Here's the drawing with two shaded views (mm, measured from the low corner). I have some questions. A direction names the side the tool comes from. Coordinates: 2 decimals unless noted, no trailing zeros. Write each loop counter-clockwise with the first axis right and the second up, starting at its lowest first coordinate (ties: lowest second). Pieces come first, ordered by that corner, then holes. Notation, with made-up numbers: M 28,75.25 L 53,75.25 A18 cw 53,96.25 Z; hole C 32.5,67 d6. An arc over 180 degrees is marked long. Answer as CSV lines item,"result". Start each with the question number.
Item 1: Suppose I cut it at B-B, the plane x = 2.5. Write out the boundary of the cut face in (y, z), and give its area (3 significant figures).
Item 2: Suppose I cut it at C-C, the plane z = 5.5. Write out the boundary of the cut face in (x, y), and give its area (3 significant figures).
Item 3: I'm going to push flat-ended pins straight in: P1, Ø1.5, axis at x = 2, z = 11.5, coming from the +Y side; P2, Ø5.5, axis at x = 7.5, y = 13, coming from the +Z side; P3, Ø5.5, axis at y = 13, z = 17, coming from the -X side. Where does each tip first touch, or does it pass through?
Item 4: Suppose I cut it at A-A, the plane y = 12.5. Write out the boundary of the cut face in (x, z), and give its area (3 significant figures).
Item 5: Suppose I cut it at D-D, the plane y = 9.5. Write out the boundary of the cut face in (x, z).
Item 6: We'd pull the mould along X, two halves only. Please class the marked faces 1, 2, 3 and 4: +X half, -X half, draft (parallel to the pull), parting line (faces both ways), or undercut.
Item 7: If I drill on line 1 along Y through (x, z) = (6.5, 20); line 2 along Z through (x, y) = (9.5, 12.5); line 3 along Z through (x, y) = (1.5, 11.25), over which ranges is the centre line in solid material (lowest first)? Write a range as [from, to].
Item 8: On a 3-axis mill with a long thin cutter (end or side, diameter ignored), from which of +Z, -Z, +X, -X, +Y, -Y can I reach the whole of each face in a straight line? I mean the marked faces 5, 6 and 7. Say none if no direction works.
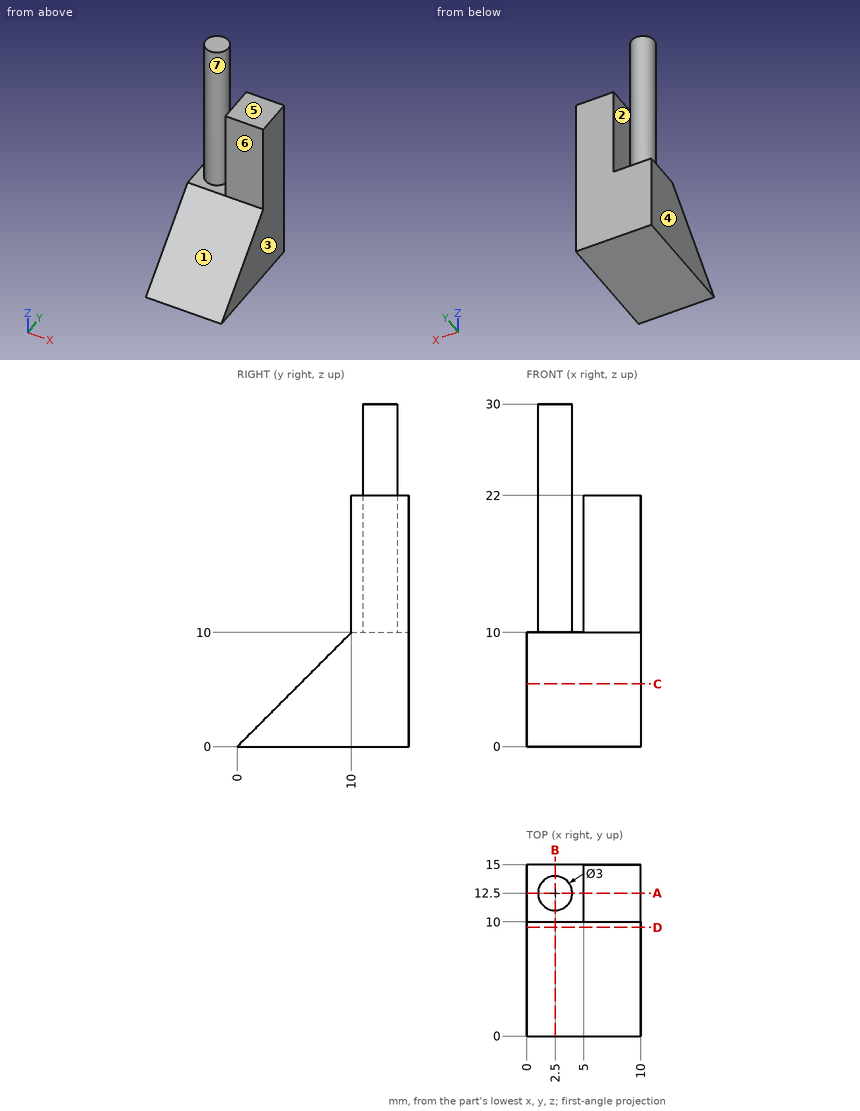
Ans:
1,outline,"M 0,0 L 15,0 L 15,10 L 14,10 L 14,30 L 11,30 L 11,10 L 10,10 Z"
1,area,"160 mm^2"
2,outline,"M 0,5.5 L 10,5.5 L 10,15 L 0,15 Z"
2,area,"95.0 mm^2"
3,P1,"stops at y = 14"
3,P2,"stops at z = 22"
3,P3,"stops at x = 1"
4,outline,"M 0,0 L 10,0 L 10,22 L 5,22 L 5,10 L 4,10 L 4,30 L 1,30 L 1,10 L 0,10 Z"
4,area,"220 mm^2"
5,outline,"M 0,0 L 10,0 L 10,9.5 L 0,9.5 Z"
6,face 1,"draft"
6,face 2,"undercut"
6,face 3,"+X half"
6,face 4,"-X half"
7,line 1,"y = [10, 15]"
7,line 2,"z = [0, 22]"
7,line 3,"z = [0, 10]"
8,face 5,"+Z, +X, +Y, -Y"
8,face 6,"+Z, +X, -X, -Y"
8,face 7,"+Z"
